from build123d import *

# Parameters (mm, degrees)
F0_R     = 3.0502649117
F0_R_2   = 1.5875
F1_DEPTH = 3.175


# Not quite as in the source:
# - a length typed as a fraction of an inch, garbled in the dataset ("3 / 203.2 mm" for 3/8 in), is restored


with BuildPart() as f1:
    # F0 (on Front) → F1 (new body)
    with BuildSketch(Plane.XZ):
        Polygon((53.3261225373, -2.7374546753), (-36.6738774627, -2.7374546753), (-36.6738774627, -15.2374546753), (53.3261225373, -15.2374546753), (83.21196348, -12.6227823928), (83.21196348, -8.9778823928), (83.21196348, -5.3521269577), align=None)
        with Locations((-30.3238774627, -8.9874546753)):
            Circle(F0_R, mode=Mode.SUBTRACT)
        with Locations((19.6761225373, -8.9874546753)):
            Circle(F0_R, mode=Mode.SUBTRACT)
        with Locations((63.21196348, -8.9778823928)):
            Circle(F0_R_2, mode=Mode.SUBTRACT)
        with Locations((73.21196348, -8.9778823928)):
            Circle(F0_R_2, mode=Mode.SUBTRACT)
    extrude(amount=F1_DEPTH)


solid = f1.part
CAD build for the part. Positions are in the model's coordinates, mm. Round coordinates to 2 decimals unless told otherwise and drop trailing zeros. Loops run counter-clockwise (first coordinate to the right, second up) from the corner with the lowest first, then second, coordinate; pieces in that order, holes last.
(1) Cut at A-A (y = -2.35). Give the cut face in (x, z) (1 decimal), plus the area to 3 significant figures.
(2) Wall check: line 1 along X through (y, z) = (-2.65, -9); line 2 along X through (y, z) = (-2.2, -8); line 3 along X through (y, z) = (-1.4, -11.75). Give the ranges that are in metal, low to high.
(3) Two-plate mould, pull along Z, no slides. Class faces 1 (the flat face through (9, -2, -2.737)), 2 (the cylindrical face through (61.626, -1.565, -8.908)), 3 (the flat face through (22, -3.175, -6)): +Z half, -Z half, draft (parallel to the pull), parting line (faces both ways), or undercut.
Findings below:
1. outline: (-36.7, -15.2) - (53.3, -15.2) - (83.2, -12.6) - (83.2, -5.4) - (53.3, -2.7) - (-36.7, -2.7) - close; hole circle Ø6.1 at (-30.3, -9); hole circle Ø6.1 at (19.7, -9); hole circle Ø3.2 at (63.2, -9); hole circle Ø3.2 at (73.2, -9)
1. area: 1,350 mm2
2. line 1: x = -36.67 to -33.37, -27.27 to 16.63, 22.73 to 61.62, 64.8 to 71.62, 74.8 to 83.21
2. line 2: x = -36.67 to -33.21, -27.44 to 16.79, 22.56 to 61.96, 64.46 to 71.96, 74.46 to 83.21
2. line 3: x = -36.67 to -31.62, -29.03 to 18.38, 20.97 to 83.21
3. face 1: +Z half
3. face 2: undercut
3. face 3: draft
